from build123d import *

# Parameters (mm, degrees)
EXTRUDE_1_DEPTH = 2
SKETCH_3_R      = 0.5
EXTRUDE_3_DEPTH = 52
SKETCH_4_R      = 0.5
EXTRUDE_4_DEPTH = 58


with BuildPart() as part:
    # Эскиз1 → Бобышка-Вытянуть1 (new body)
    with BuildSketch(Plane(origin=(0, 0, 0), x_dir=(0, 0, -1), z_dir=(1, 0, 0))):
        Polygon((-25, 6), (-22.034972426, 6), (-13.466084386, 0), (0, 0), (0, 58), (-25, 58), align=None)
    extrude(amount=EXTRUDE_1_DEPTH)

    # Эскиз3 → Бобышка-Вытянуть3 (add)
    with BuildSketch(Plane.XZ.offset(-6)):
        with BuildLine():
            Line((0, 25), (0, 26))
            ThreePointArc((0, 26), (1, 27), (2, 26))
            Line((2, 26), (2, 25))
            Line((2, 25), (0, 25))
        make_face()
        with Locations(Location((1, 26, 0), (0, 0, 270))):
            Circle(SKETCH_3_R, mode=Mode.SUBTRACT)
    extrude(amount=-EXTRUDE_3_DEPTH)

    # Эскиз4 → Бобышка-Вытянуть4 (add)
    with BuildSketch(Plane(origin=(0, 0, 0), x_dir=(1, 0, 0), z_dir=(0, 1, 0))):
        with BuildLine():
            Line((3, 0), (2, 0))
            Line((2, 0), (2, -2))
            Line((2, -2), (3, -2))
            ThreePointArc((3, -2), (4, -1), (3, 0))
        make_face()
        with Locations(Location((3, -1, 0), (0, 0, 90))):
            Circle(SKETCH_4_R, mode=Mode.SUBTRACT)
    extrude(amount=EXTRUDE_4_DEPTH)


solid = part.part
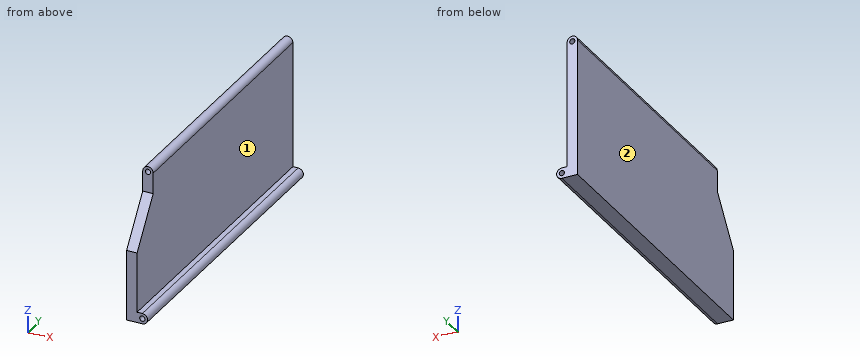
Check sheet for the modelled part. Datum: model origin and axes. Units: mm. Face numbers are marked on the shaded views. A direction names the side the tool comes from. Coordinates: 2 decimals unless noted, no trailing zeros. Write each loop counter-clockwise with the first axis right and the second up, starting at its lowest first coordinate (ties: lowest second). Pieces come first, ordered by that corner, then holes. Notation, with made-up numbers: M -5.5,59.5 L 38.5,59.5 A28 cw 38.5,96.5 Z; hole C -6.75,-14.75 d7. An arc over 180 degrees is marked long. Answer as CSV lines item,"result".
Q1. Set-up check for the marked faces 1 and 2: record each of +Z, -Z, +X, -X, +Y, -Y from which the full face is reachable in a straight line by a thin tool's end or side.
Check result:
face 1,"+Z, +X, +Y, -Y"
face 2,"+Z, -Z, -X, +Y, -Y"
Q2. Material ranges on probe 1 along X at (y, z) = (42.5, 26); probe 2 along X at (y, z) = (42.5, 1), recorded low to high. Write a range as from..to.
Check result:
probe 1,"0..0.5, 1.5..2"
probe 2,"0..2.5, 3.5..4"
Q3. Cross-section at A-A (y = 25). Record the boundary of the cut face in (x, z), then the cut area to 3 significant figures.
Check result:
outline,"M 0,0 L 3,0 A1 ccw 3,2 L 2,2 L 2,26 A1 ccw 0,26 Z; hole C 1,26 d1; hole C 3,1 d1"
area,"55.6 mm^2"
Q4. Cross-section at B-B (z = 5.5). Record the boundary of the cut face in (x, y), then the cut area to 3 significant figures.
Check result:
outline,"M 0,0 L 2,0 L 2,58 L 0,58 Z"
area,"116 mm^2"
Q5. Go/stop test with flat-tipped pins: pin 1 (8 mm diameter, centred on y = 37, z = 12, fed in from +X); pin 2 (0.5 mm diameter, centred on x = 2.5, y = 16, fed in from +Z); pin 3 (1.6 mm diameter, centred on x = 1.5, z = 23.5, fed in from -Y). Record where each tip stops, or that it passes through.
Check result:
pin 1,"x = 2"
pin 2,"z = 2"
pin 3,"y = 6"
Q6. Cross-section at C-C (z = 20.5). Record the boundary of the cut face in (x, y).
Check result:
outline,"M 0,4.93 L 2,4.93 L 2,58 L 0,58 Z"
